Verification items for the finished model (mm, model axes). A direction names the side the tool comes from. Coordinates: 2 decimals unless noted, no trailing zeros. Order: outer loops, then holes, each group sorted by start corner. A loop starts at its lowest first (then second) coordinate and runs counter-clockwise, first axis right, second up. Notation, with made-up numbers: (-3.75, -13.5) -> (1.25, -13.5) arc R21 ccw to (1.25, 1.5) -> close; hole circle Ø9 at (-28.5, 37). An arc over 180 degrees is marked (long way). Use CSV: the item, a comma, the result in double quotes. Start each with the question number.
1) Scan lines: line 1 along Y through (x, z) = (-15, -5.75); line 2 along Z through (x, y) = (11, -8); line 3 along X through (y, z) = (-0.25, -4.25). Record each from-to range of solid material in increasing order.
2) Go/stop test with flat-tipped pins: pin 1 (2 mm diameter, centred on x = 11.5, y = -6, fed in from -Z); pin 2 (9 mm diameter, centred on x = -8, y = -3.5, fed in from -Z); pin 3 (9 mm diameter, centred on x = -15, y = -4, fed in from +Z); pin 4 (2.5 mm diameter, centred on y = 2.5, z = -6, fed in from -X). Record where each tip stops, or that it passes through.
3) Sectioned sample at C-C on y = 0. Give the number of separate pieces and of enclosed holes in the cut face, then the cut area to 3 significant figures.
4) Release check for a two-part mould opening along Y. For faces 5 (the flat face through (-9.4, -9.5, 4.5)), 6 (the flat face through (-9.6, 9.5, -6.5)), 7 (the cylindrical face through (17.5, -0.1, 5.5)) record: released by +Y, released by -Y, zero draft, split by the parting line, or undercut.
5) Sectioned sample at A-A on z = 1.5. Record the boundary of the cut face in (x, y), then the cut area to 3 significant figures.
6) Sectioned sample at B-B on z = 5.5. Record the boundary of the cut face in (x, y).
7) Tool access check on faces 1 (the flat face through (-4.5, -9.5, -0.1)), 2 (the flat face through (-9.6, 9.5, 6.5)), 3 (the flat face through (9.4, -9.5, 4.5)), 4 (the flat face through (12, 0, -7)). Record the directions out of +Z, -Z, +X, -X, +Y, -Y that give a thin tool (end or side, any length) a straight path to the whole face; none if there is none.
from build123d import *

# Parameters (mm, degrees)
BOSS_EXTRUDE1_DEPTH = 10
CUT_EXTRUDE1_DEPTH  = 4
CUT_EXTRUDE2_START  = -7
CUT_EXTRUDE2_DEPTH  = 7
CUT_EXTRUDE3_START  = 14
CUT_EXTRUDE3_DEPTH  = 7
SKETCH3_R           = 2.5
CUT_EXTRUDE4_DEPTH  = 10
CHAMFER2_SIZE       = 1
CHAMFER3_SIZE       = 1
CHAMFER4_SIZE       = 1
SHELL1_START        = -4
SHELL1_OUTLINE_W    = 10
SHELL1_OUTLINE_H    = 14
SHELL1_DEPTH        = 8
SHELL1_START_2      = -7
SHELL1_2_OUTLINE_W  = 4
SHELL1_2_OUTLINE_H  = 14
SHELL1_2_DEPTH      = 14
CHAMFER5_SIZE       = 1


# Read off the part's stored shape, not the designer's step: Shell1
with BuildPart() as part:
    # Sketch1 → Boss-Extrude1 (new, symmetric)
    with BuildSketch(Plane.XY):
        with BuildLine():
            Line((-15, 10), (15, 10))
            ThreePointArc((15, 10), (25, 0), (15, -10))
            Line((15, -10), (-15, -10))
            ThreePointArc((-15, -10), (-25, 0), (-15, 10))
        make_face()
    extrude(amount=BOSS_EXTRUDE1_DEPTH, both=True)

    # Sketch2 → Cut-Extrude1 (cut, symmetric)
    with BuildSketch(Plane.XY):
        with BuildLine():
            Line((-15, 10), (-5, 10))
            Line((-5, 10), (-5, -10))
            Line((-5, -10), (-15, -10))
            ThreePointArc((-15, -10), (-25, 0), (-15, 10))
        make_face()
        with BuildLine():
            Line((5, -10), (15, -10))
            ThreePointArc((15, -10), (25, 0), (15, 10))
            Line((15, 10), (5, 10))
            Line((5, 10), (5, -10))
        make_face()
    extrude(amount=CUT_EXTRUDE1_DEPTH, both=True, mode=Mode.SUBTRACT)

    # Sketch2<2> → Cut-Extrude2 (cut)
    with BuildSketch(Plane.XY.offset(CUT_EXTRUDE2_START)):
        with BuildLine():
            Line((-15, 10), (-5, 10))
            Line((-5, 10), (-5, -10))
            Line((-5, -10), (-15, -10))
            ThreePointArc((-15, -10), (-25, 0), (-15, 10))
        make_face()
        with BuildLine():
            Line((5, -10), (15, -10))
            ThreePointArc((15, -10), (25, 0), (15, 10))
            Line((15, 10), (5, 10))
            Line((5, 10), (5, -10))
        make_face()
    extrude(amount=-CUT_EXTRUDE2_DEPTH, mode=Mode.SUBTRACT)

    # Sketch2<3> → Cut-Extrude3 (cut)
    with BuildSketch(Plane.XY.offset(CUT_EXTRUDE3_START)):
        with BuildLine():
            Line((-15, 10), (-5, 10))
            Line((-5, 10), (-5, -10))
            Line((-5, -10), (-15, -10))
            ThreePointArc((-15, -10), (-25, 0), (-15, 10))
        make_face()
        with BuildLine():
            Line((5, -10), (15, -10))
            ThreePointArc((15, -10), (25, 0), (15, 10))
            Line((15, 10), (5, 10))
            Line((5, 10), (5, -10))
        make_face()
    extrude(amount=-CUT_EXTRUDE3_DEPTH, mode=Mode.SUBTRACT)

    # Sketch3 → Cut-Extrude4 (cut, symmetric)
    with BuildSketch(Plane.XY):
        with Locations((-15, 0)):
            Circle(SKETCH3_R)
        with Locations(Location((15, 0, 0), (0, 0, 180))):
            Circle(SKETCH3_R)
    extrude(amount=CUT_EXTRUDE4_DEPTH, both=True, mode=Mode.SUBTRACT)

    # Chamfer2
    chamfer2_edges = [part.edges().sort_by_distance(p)[0] for p in [
        (10, -10, 7),
        (-25, 0, -4),
        (-10, 10, -4),
        (-10, -10, -4),
        (-25, 0, 4),
        (-10, -10, 4),
        (-10, 10, 4),
        (25, 0, -4),
        (10, -10, -4),
        (10, 10, -4),
        (25, 0, 4),
        (10, 10, 4),
        (10, -10, 4),
        (-25, 0, -7),
        (-10, -10, -7),
        (-10, 10, -7),
        (25, 0, -7),
        (10, 10, -7),
        (10, -10, -7),
        (-25, 0, 7),
        (-10, -10, 7),
        (-10, 10, 7),
        (25, 0, 7),
        (10, 10, 7),
    ]]
    chamfer(chamfer2_edges, length=CHAMFER2_SIZE)

    # Chamfer3
    chamfer3_edges = [part.edges().sort_by_distance(p)[0] for p in [
        (-5, -10, -8),
        (5, -10, -8),
        (5, -10, 8),
        (-5, -10, 8),
        (-5, 10, 8),
        (5, 10, 8),
        (5, 10, -8),
        (-5, 10, -8),
    ]]
    chamfer(chamfer3_edges, length=CHAMFER3_SIZE)

    # Chamfer4
    chamfer4_edges = [part.edges().sort_by_distance(p)[0] for p in [
        (-5, 0, -10),
        (0, -10, 10),
        (0, -10, -10),
        (0, 10, -10),
        (5, 0, -10),
        (-4.5, 9.5, -10),
        (4.5, 9.5, -10),
        (4.5, -9.5, -10),
        (-4.5, -9.5, -10),
        (5, 0, 10),
        (0, 10, 10),
        (-5, 0, 10),
        (4.5, 9.5, 10),
        (-4.5, 9.5, 10),
        (-4.5, -9.5, 10),
        (4.5, -9.5, 10),
    ]]
    chamfer(chamfer4_edges, length=CHAMFER4_SIZE)

    # Shell1 outline → Shell1 (cut)
    with BuildSketch(Plane.XY.offset(SHELL1_START)):
        Rectangle(SHELL1_OUTLINE_W, SHELL1_OUTLINE_H)
    extrude(amount=SHELL1_DEPTH, mode=Mode.SUBTRACT)

    # Shell1 2 outline → Shell1 2 (cut)
    with BuildSketch(Plane.XY.offset(SHELL1_START_2)):
        Rectangle(SHELL1_2_OUTLINE_W, SHELL1_2_OUTLINE_H)
    extrude(amount=SHELL1_2_DEPTH, mode=Mode.SUBTRACT)

    # Chamfer5
    chamfer5_edges = [part.edges().sort_by_distance(p)[0] for p in [
        (5, -10, 0),
        (-5, -10, 0),
        (5, 10, 0),
        (-5, 10, 0),
    ]]
    chamfer(chamfer5_edges, length=CHAMFER5_SIZE)


solid = part.part
Answers follow:
1,line 1,"y = -10 to -2.5, 2.5 to 10"
1,line 2,"z = -7 to -4, 4 to 7"
1,line 3,"x = -24.25 to -17.49, -12.51 to -2, 2 to 12.51, 17.49 to 24.25"
2,pin 1,"stops at z = -7"
2,pin 2,"stops at z = -10"
2,pin 3,"stops at z = 7"
2,pin 4,"stops at x = -24.92"
3,separate pieces,"6"
3,enclosed holes,"0"
3,area,"270 mm²"
4,face 5,"released by -Y"
4,face 6,"released by +Y"
4,face 7,"undercut"
5,outline,"(-5, -9) -> (-4, -10) -> (4, -10) -> (5, -9) -> (5, -7) -> (-5, -7) -> close; (-5, 7) -> (5, 7) -> (5, 9) -> (4, 10) -> (-4, 10) -> (-5, 9) -> close"
5,area,"58.0 mm²"
6,outline,"(-15, -10) -> (15, -10) arc R10 ccw to (15, 10) -> (-15, 10) arc R10 ccw to start; hole circle Ø5 at (-15, 0); hole (-2, -7) -> (2, -7) -> (2, 7) -> (-2, 7) -> close; hole circle Ø5 at (15, 0)"
7,face 1,"-X, -Y"
7,face 2,"+Z, -X, +Y"
7,face 3,"+X, -Y"
7,face 4,"-Z, +X, +Y, -Y"
